Autodesk Inventor part; units mm, degrees
ref_plane "YZ Plane" through (0, 0, 0) normal (1, 0, 0) x (0, 1, 0)
ref_plane "XZ Plane" through (0, 0, 0) normal (0, 1, 0) x (-1, 0, 0)
ref_plane "XY Plane" through (0, 0, 0) normal (0, 0, 1) x (1, 0, 0)
sketch "Sketch1" plane through (0, 0, 0) normal (0, 0, 1) x (1, 0, 0)
  line L0 (0, 0) -> (19, 0)
  line L1 (19, 0) -> (19, 9)
  line L2 (19, 9) -> (0, 9)
  line L3 (0, 9) -> (0, 0)
  point P0 (9.5, 9)
  dimension "d0" = 19
  dimension "d1" = 9
extrude "Extrusion1" add sketch "Sketch1" along normal blind 3
sketch "Sketch10" plane through (0, 0, 0) normal (-1, 0, 0) x (0, 0, 1)
  line L0 (0, 0) -> (3, 0)
  line L1 (3, 9) -> (3, 0)
  line L2 (3, 0) -> (2, 0)
  line L3 (2, 0) -> (2, 6)
  line L4 (2, 6) -> (3, 6)
  line L5 (3, 6) -> (3, 0)
  line L6 (3, 0) -> (2, 1)
  line L7 (3, 0) -> (4.4142, 0) construction
  line L8 (2, 1) -> (3, 2)
  line L9 (3, 0) -> (3, 9)
  line L10 (3, 2) -> (2, 3)
  line L11 (2, 3) -> (3, 4)
  line L12 (2, 5) -> (3, 4)
  line L13 (2, 5) -> (3, 5)
  dimension "d23" = 1
  dimension "d24" = 6
  dimension "d25" = 135
  dimension "d26" = 90
extrude "Extrusion8" cut sketch "Sketch10" against normal up to next contours L6 L8 L1 | L10 L11 L1 | L12 L13 L1 | L3 L4 L1 L13
sketch "Sketch12" plane through (0, 0, 3) normal (0, 0, 1) x (1, 0, 0)
  line L0 (19, 9) -> (0, 9)
  line L1 (11.5494, 5.95) -> (7.4494, 5.95)
  line L2 (7.4494, 5.95) -> (7.4494, 8.05)
  line L3 (7.4494, 8.05) -> (11.5494, 8.05)
  line L4 (11.5494, 8.05) -> (11.5494, 5.95)
  line L5 (11.5494, 5.95) -> (7.4494, 8.05) construction
  line L6 (7.4494, 5.95) -> (11.5494, 8.05) construction
  line L7 (10.5494, 7.1) -> (8.4494, 7.1)
  line L8 (8.4494, 7.1) -> (8.4494, 9)
  line L9 (8.4494, 9) -> (10.5494, 9)
  line L10 (10.5494, 9) -> (10.5494, 7.1)
  line L11 (10.5494, 7.1) -> (8.4494, 9) construction
  line L12 (8.4494, 7.1) -> (10.5494, 9) construction
  point P0 (0, 0)
  point P1 (9.4994, 7)
  point P2 (9.4994, 8.05)
  dimension "d47" = 2
  dimension "d48" = 4.1
  dimension "d49" = 2.1
  dimension "d50" = 2.1
extrude "Extrusion10" cut sketch "Sketch12" against normal up to next
sketch "Sketch14" plane through (0, 0, 2) normal (0, 0, 1) x (1, 0, 0)
  line L0 (6.4994, 5) -> (12.4994, 5)
  line L1 (12.4994, 5) -> (12.4994, 6)
  line L2 (12.4994, 6) -> (6.4994, 6)
  line L3 (6.4994, 6) -> (6.4994, 5)
  line L4 (6.4994, 5) -> (12.4994, 6) construction
  line L5 (12.4994, 5) -> (6.4994, 6) construction
  line L6 (19, 9) -> (10.5494, 9)
  point P0 (0, 0)
  point P1 (9.4994, 5.5)
  dimension "d57" = 6
  dimension "d58" = 1
  dimension "d59" = 3.5
extrude "Extrusion12" add sketch "Sketch14" along normal blind 1
chamfer "Chamfer1" distance 0.5 angle 45 1 edges at (9.4994, 5, 3)
sketch "Sketch16" plane through (0, 0, 0) normal (0, 0, -1) x (-1, 0, 0)
  line L0 (-11.5494, 8.05) -> (-11.5494, 6)
  line L1 (-10.5494, 8.05) -> (-11.5494, 8.05)
  arc A0 (-11.5494, 8.05) -> (-10.5494, 8.05) centre (-11.0494, 8.916) ccw
  line L2 (-8.4494, 8.05) -> (-7.4494, 8.05)
  arc A1 (-8.4494, 8.05) -> (-7.4494, 8.05) centre (-7.9494, 8.916) ccw
  point P0 (0, 0)
  dimension "d66" = 1
  dimension "d67" = 1
extrude "Extrusion13" add sketch "Sketch16" against normal up to surface (3 mm away)
sketch "Sketch18" plane through (0, 0, 0) normal (0, -1, 0) x (1, 0, 0)
  line L0 (9.5, 3) -> (8.5, 2)
  line L1 (9.5, 3) -> (10.9142, 3) construction
  line L2 (8.5, 2) -> (7.5, 3)
  line L3 (7.5, 3) -> (6.4994, 2)
  line L4 (6.4994, 2) -> (5.5, 3)
  line L5 (5.5, 3) -> (4.5, 2)
  line L6 (5.5, 3) -> (6.9142, 3) construction
  line L7 (4.5, 2) -> (3.5, 3)
  line L8 (3.5, 3) -> (2.5, 2)
  line L9 (0, 3) -> (6.4994, 3)
  line L10 (0, 3) -> (3.5, 3)
  line L11 (19, 3) -> (19, 2)
  line L12 (19, 2) -> (16.5, 2)
  line L13 (0, 2) -> (0, 3)
  line L14 (8.5, 2) -> (6.4994, 2)
  line L15 (6.4994, 2) -> (4.5, 2)
  line L16 (4.5, 2) -> (2.5, 2)
  line L17 (3.5, 3) -> (5.5, 3)
  line L18 (5.5, 3) -> (7.5, 3)
  line L19 (7.5, 3) -> (9.5, 3)
  line L20 (2.5, 2) -> (0, 2)
  line L21 (9.5, 2.2481) -> (9.5, 2.7918)
  line L22 (9.5, 3) -> (10.5, 2)
  line L23 (10.5, 2) -> (11.5, 3)
  line L24 (11.5, 3) -> (12.5006, 2)
  line L25 (12.5006, 2) -> (13.5, 3)
  line L26 (13.5, 3) -> (14.5, 2)
  line L27 (14.5, 2) -> (15.5, 3)
  line L28 (15.5, 3) -> (16.5, 2)
  line L29 (14.5, 2) -> (12.5006, 2)
  line L30 (16.5, 2) -> (14.5, 2)
  line L31 (12.5006, 2) -> (10.5, 2)
  line L32 (10.5, 2) -> (8.5, 2)
  line L33 (11.5, 3) -> (13.5, 3)
  line L34 (13.5, 3) -> (15.5, 3)
  line L35 (15.5, 3) -> (19, 3)
  line L36 (9.5, 3) -> (11.5, 3)
  point P0 (0, 0)
  dimension "d71" = 135
  dimension "d72" = 90
  dimension "d73" = 135
extrude "Extrusion14" cut sketch "Sketch18" against normal blind 5 contours L0 L2 L19 | L36 L23 L22 | L3 L4 L9 L18 | L33 L25 L24 | L34 L27 L26 | L5 L7 L9 | L35 L11 L12 L28 | L8 L20 L13 L9
properties part number "Clamp-part2(moving)-Base9x19mm."
The listing builds one solid part. Answer for the finished solid, in the listing's coordinates (mm). A direction names the side the tool comes from. Round coordinates to 2 decimals unless told otherwise and drop trailing zeros. Loops run counter-clockwise (first coordinate to the right, second up) from the corner with the lowest first, then second, coordinate; pieces in that order, holes last. Notation, with made-up numbers: (41.25, 20.25) - (88.25, 20.25) arc R37 ccw to (88.25, 59.25) - close; hole circle Ø2 at (-13, 23.25). An arc over 180 degrees is marked (long way). Return JSON: item names as keys, results as strings. Group by question number.
1. The part is cut by section A-A on y = 8.75. Determine the outline of the cut face in (x, z).
2. The part is cut by section D-D on y = 5.75. Determine the outline of the cut face in (x, z), then the cut area to 3 significant figures.
3. Each of these flat-tipped pins is pushed along its axis until it touches: P1, Ø0.5, axis at y = 5.5, z = 2.5, coming from the -X side; P2, Ø0.5, axis at x = 16.5, z = 2.5, coming from the -Y side; P3, Ø0.8, axis at x = 9.5, z = 2.5, coming from the +Y side. Where does it stop, or does it pass through?
4. The mould has two halves that part along X. Classify faces 1 (the flat face through (15.5, 4.6, 2.4)), 2 (the flat face through (12.1, 4, 2.4)): pulls with the +X half, pulls with the -X half, needs draft (parallel to the pull), parting line crosses it, or undercut.
5. The part is cut by section B-B on z = 1.25. Determine the outline of the cut face in (x, y).
6. Consider probe 1 along X at (y, z) = (8.5, 2.4); probe 2 along X at (y, z) = (7.5, 1.4); probe 3 along Y at (x, z) = (1, 2.8). Determine where each line is inside the solid, lowest interval first.
7. The part is cut by section C-C on x = 4.75. Determine the outline of the cut face in (y, z).
8. Which of the six approach directions +Z, -Z, +X, -X, +Y, -Y give full straight-line access (tool end or side, diameter ignored) to faces 3 (the flat face through (9.4, 5.7, 3)), 4 (the flat face through (9.5, 6, 2.5)), 5 (the flat face through (14.1, 2, 2.4)), 6 (the flat face through (11.5, 1.4, 2.4))?
Resolved:
{
 "1": {"outline": "(0, 0) - (8.45, 0) - (8.45, 3) - (0, 3) - close; (10.55, 0) - (19, 0) - (19, 3) - (10.55, 3) - close"},
 "2": {"outline": "(0, 0) - (19, 0) - (19, 2) - (12.5, 2) - (12.5, 3) - (6.5, 3) - (6.5, 2) - (0, 2) - close", "area": "44.0 mm²"},
 "3": {"P1": "stops at x = 6.5", "P2": "stops at y = 6", "P3": "stops at y = 6"},
 "4": {"face 1": "needs draft", "face 2": "undercut"},
 "5": {"outline": "(0, 0) - (19, 0) - (19, 9) - (10.55, 9) - (10.55, 8.05) arc R1 ccw to (11.55, 8.05) - (11.55, 5.95) - (7.45, 5.95) - (7.45, 8.05) arc R1 ccw to (8.45, 8.05) - (8.45, 9) - (0, 9) - close"},
 "6": {"probe 1": "x = 0 to 8.45, 10.55 to 19", "probe 2": "x = 0 to 7.45, 11.55 to 19", "probe 3": "y = 6 to 9"},
 "7": {"outline": "(0, 0) - (9, 0) - (9, 3) - (6, 3) - (6, 2) - (5, 2) - (4.75, 2.25) - (3.25, 2.25) - (3, 2) - (2.75, 2.25) - (1.25, 2.25) - (1, 2) - (0.75, 2.25) - (0, 2.25) - close"},
 "8": {"face 3": "+Z, +X, -X, +Y, -Y", "face 4": "+Z, -Z", "face 5": "+Z, -Y", "face 6": "+Z, +X, -X"}
}
